The drawing under review shows one solid part. Ordinate dimensions are in mm from its lowest x, y, z. Round coordinates to 2 decimals unless told otherwise and drop trailing zeros. Order: outer loops, then holes, each group sorted by start corner. A loop starts at its lowest first (then second) coordinate and runs counter-clockwise, first axis right, second up. Notation, with made-up numbers: M -16.75,62.5 L 2.25,62.5 A16 cw 2.25,74.5 Z; hole C 57.5,7.5 d2. An arc over 180 degrees is marked long. Answer as a JSON object with one key per item and string values.
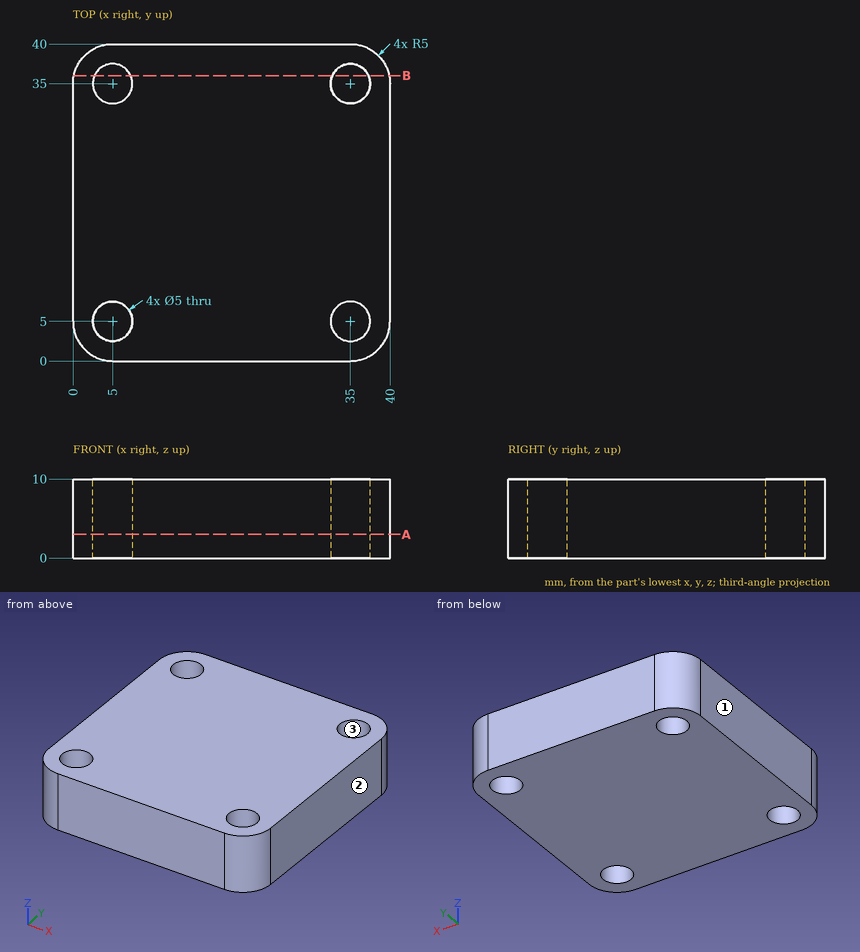
1) For L1, parallel to Y at x = 35, z = 2.5, list the stretches that pass through material, from the lowest coordinate up.
Geometry check:
{"L1": "y = 0 to 2.5, 7.5 to 32.5, 37.5 to 40"}
2) Mouldability with a two-part tool opening along X and no side actions: class the marked faces 1, 2 and 3 as +X half, -X half, draft (parallel to the pull), parting line (faces both ways), or undercut.
Geometry check:
{"face 1": "-X half", "face 2": "+X half", "face 3": "undercut"}
3) Add section B-B on y = 36. State the section outline as (x, z) points, and give its area (3 significant figures).
Geometry check:
{"outline": "M 0.1,0 L 2.71,0 L 2.71,10 L 0.1,10 Z; M 7.29,0 L 32.71,0 L 32.71,10 L 7.29,10 Z; M 37.29,0 L 39.9,0 L 39.9,10 L 37.29,10 Z", "area": "306 mm²"}
4) Add section A-A on z = 3. State the section outline as (x, y) points.
Geometry check:
{"outline": "M 0,5 A5 ccw 5,0 L 35,0 A5 ccw 40,5 L 40,35 A5 ccw 35,40 L 5,40 A5 ccw 0,35 Z; hole C 5,5 d5; hole C 5,35 d5; hole C 35,5 d5; hole C 35,35 d5"}
